```python
from build123d import *

# Parameters (mm, degrees)
F1_DEPTH = 25.4
F3_DEPTH = 12.7
F5_DEPTH = 31.75
F6_DEPTH = 12.7
F8_DEPTH = 12.7
F9_DEPTH = 25.4


with BuildPart() as f1:
    # F0 (on Right) → F1 (new body)
    with BuildSketch(Plane.YZ):
        Polygon((0, 31.75), (0, 0), (31.75, 0), (19.05, 31.75), align=None)
        Polygon((19.05, 31.75), (31.75, 0), (57.15, 0), (57.15, 31.75), align=None)
    extrude(amount=F1_DEPTH)

    # F2 (on face) → F3 (cut)
    with BuildSketch(Plane.YZ.offset(25.4)):
        Polygon((57.15, 31.75), (19.05, 31.75), (31.75, 0), (57.15, 0), align=None)
    extrude(amount=-F3_DEPTH, mode=Mode.SUBTRACT)

    # F5 (add): faces of the model
    f5_faces = [f1.faces().sort_by_distance(p)[0] for p in [
        (12.7, 41.0633333333, 16.9333333333),
        (25.4, 12.9645833333, 14.5520833333),
    ]]
    extrude(f5_faces, amount=F5_DEPTH)

    # F4 (on face) → F6 (cut)
    with BuildSketch(Plane(origin=(0, 0, 0), x_dir=(0, -1, 0), z_dir=(-1, 0, 0))):
        Polygon((-57.15, 31.75), (-57.15, 0), (-36.5937203169, 0), (-19.05, 31.75), align=None)
    extrude(amount=-F6_DEPTH, mode=Mode.SUBTRACT)

    # F7 (on face) → F8 (cut)
    with BuildSketch(Plane.YZ.offset(44.45)):
        Polygon((57.15, 31.75), (44.45, 31.75), (57.15, 0), align=None)
    extrude(amount=-F8_DEPTH, mode=Mode.SUBTRACT)

    # F9 (cut): a face of the model
    f9_faces = [f1.faces().sort_by_distance(p)[0] for p in [
        (31.75, 52.9166666667, 21.1666666667),
    ]]
    extrude(f9_faces, amount=-F9_DEPTH, mode=Mode.SUBTRACT)


solid = f1.part
```
Geometry: final body of the model. Coordinates: model frame, mm. A direction names the side the tool comes from. Coordinates: 2 decimals unless noted, no trailing zeros. Order: outer loops, then holes, each group sorted by start corner. A loop starts at its lowest first (then second) coordinate and runs counter-clockwise, first axis right, second up. Notation, with made-up numbers: M -13,89.25 L 17,89.25 A7 cw 17,100.25 Z; hole C 49.5,-21.5 d1. An arc over 180 degrees is marked long. Answer in a Markdown table with one row per item. Add a question column.
Q1. Section query B-B on x = 53.5. Return the cut outline in (y, z).
Q2. Section query A-A on z = 15. Return the cut outline in (x, y).
Q3. Line query: L1, parallel to X at y = 39, z = 28; L2, parallel to Y at x = 3.5, z = 8; L3, parallel to Y at x = 6.5, z = 13. Output: solid intervals per line, ascending.
Q4. Section query D-D on z = 4.5. Return the cut outline in (x, y).
Q5. Contact query for flat-ended pins moving along their axis: P1, Ø10, axis at y = 15, z = 26, coming from the -X side; P2, Ø8, axis at x = 20, z = 19.5, coming from the +Y side; P3, Ø4, axis at y = 43, z = 14, coming from the +X side. Output: stop coordinate, or through.
Q6. Reachability of faces 1 (the flat face through (12.7, 38, 16)), 2 (the flat face through (0, 14, 16)), 3 (the flat face through (44.45, 38, 16)) from +Z, -Z, +X, -X, +Y, -Y: full face, straight path, thin tool, end or side. Return the list, or none.
Q7. Section query C-C on y = 41.5. Return the cut outline in (x, z).
Completed:
| question | item | result |
|---|---|---|
| 1 | outline | M 0,0 L 31.75,0 L 19.05,31.75 L 0,31.75 Z |
| 2 | outline | M 0,0 L 57.15,0 L 57.15,25.75 L 44.45,25.75 L 44.45,51.15 L 12.7,51.15 L 12.7,28.31 L 0,28.31 Z |
| 3 | L1 | x = 12.7 to 44.45 |
| 3 | L2 | y = 0 to 32.17 |
| 3 | L3 | y = 0 to 29.41 |
| 4 | outline | M 0,0 L 57.15,0 L 57.15,29.95 L 44.45,29.95 L 44.45,55.35 L 12.7,55.35 L 12.7,34.11 L 0,34.11 Z |
| 5 | P1 | stops at x = 0 |
| 5 | P2 | stops at y = 50.95 |
| 5 | P3 | stops at x = 44.45 |
| 6 | face 1 | +Z, -X, +Y |
| 6 | face 2 | +Z, -Z, -X, +Y, -Y |
| 6 | face 3 | +Z, +X, +Y |
| 7 | outline | M 12.7,0 L 44.45,0 L 44.45,31.75 L 12.7,31.75 Z |
